Check sheet for the modelled part. Datum: model origin and axes. Units: mm. Round coordinates to 2 decimals unless told otherwise and drop trailing zeros. Write each loop counter-clockwise with the first axis right and the second up, starting at its lowest first coordinate (ties: lowest second). Pieces come first, ordered by that corner, then holes.
Item 1: Cross-section at B-B on x = 111.5. Enter the section's corners in (y, z), plus the area to 3 significant figures.
Item 2: Cross-section at A-A on z = -2.5. Count the separate pieces of the cut face and the enclosed holes in it, plus the area to 3 significant figures.
Item 3: Material ranges on line 1 (Y direction, x = 19, z = -1.5); line 2 (X direction, y = 9, z = -1.9); line 3 (Y direction, x = 10, z = -1.6), recorded low to high.
Item 4: Go/stop test with flat-tipped pins: pin 1 Ø2 at (y, z) = (11.5, -2.5) entering from -X; pin 2 Ø1.5 at (x, z) = (74.5, -1) entering from +Y; pin 3 Ø3 at (x, y) = (10, 0) entering from -Z; pin 4 Ø2 at (y, z) = (-12, -1) entering from +X. Record where each tip stops, or that it passes through.
from build123d import *

# Parameters (mm, degrees)
BRIDA_BASE1_DEPTH     = 4
CROQUIS6_R            = 1.2
CORTAR_EXTRUIR1_DEPTH = 361.432850889
TALADRO_ROSCADO_M3_D  = 2.5
CROQUIS11_R           = 1.7
CORTAR_EXTRUIR2_DEPTH = 361.432850889
REDONDEO1_START       = -5
REDONDEO1_DEPTH       = 6
REDONDEO1_START_2     = -4
REDONDEO1_2_DEPTH     = 4
REDONDEO2_R           = 0.5


with BuildPart() as part:
    # Brida base1: sheet metal written as solids
    # Croquis1 → Brida base1 (new body)
    with BuildSketch(Plane.XY):
        Polygon((0, -4.1), (0, 4.1), (8, 4.1), (15.8, 4.1), (15.8, 17.2), (22.2, 17.2), (22.2, 4.1), (176.8, 4.1), (176.8, 17.2), (183.2, 17.2), (183.2, 4.1), (337.8, 4.1), (337.8, 17.2), (344.2, 17.2), (344.2, 4.1), (352, 4.1), (360, 4.1), (360, -4.1), (352, -4.1), (344.2, -4.1), (344.2, -17.2), (337.8, -17.2), (337.8, -4.1), (183.2, -4.1), (183.2, -17.2), (176.8, -17.2), (176.8, -4.1), (22.2, -4.1), (22.2, -17.2), (15.8, -17.2), (15.8, -4.1), (8, -4.1), align=None)
    extrude(amount=-BRIDA_BASE1_DEPTH)

    # Croquis6 → Cortar-Extruir1 (cut, through all)
    with BuildSketch(Plane.XY):
        with Locations((10, 0)):
            Circle(CROQUIS6_R)
        with Locations((350, 0)):
            Circle(CROQUIS6_R)
        with Locations((170, 0)):
            Circle(CROQUIS6_R)
    extrude(amount=-CORTAR_EXTRUIR1_DEPTH, mode=Mode.SUBTRACT)

    # Taladro roscado M3 (through all)
    with Locations(Plane.XY):
        with Locations((10, 0), (170, 0), (350, 0)):
            Hole(TALADRO_ROSCADO_M3_D / 2)

    # Croquis11 → Cortar-Extruir2 (cut, through all)
    with BuildSketch(Plane.XY):
        with Locations((19, 14)):
            Circle(CROQUIS11_R)
        with Locations((180, 14)):
            Circle(CROQUIS11_R)
        with Locations((341, 14)):
            Circle(CROQUIS11_R)
        with Locations(Location((341, -14, 0), (0, 0, 180))):
            Circle(CROQUIS11_R)
        with Locations(Location((180, -14, 0), (0, 0, 180))):
            Circle(CROQUIS11_R)
        with Locations(Location((19, -14, 0), (0, 0, 180))):
            Circle(CROQUIS11_R)
    extrude(amount=-CORTAR_EXTRUIR2_DEPTH, mode=Mode.SUBTRACT)

    # Redondeo1: read off the stored shape, not the designer's step
    # Redondeo1 outline → Redondeo1 (cut)
    with BuildSketch(Plane.XY.offset(REDONDEO1_START)):
        with BuildLine():
            ThreePointArc((15.8, 14), (16.7372583, 16.2627417), (19, 17.2))
            Line((19, 17.2), (15.8, 17.2))
            Line((15.8, 17.2), (15.8, 14))
        make_face()
        with BuildLine():
            ThreePointArc((19, 17.2), (21.2627417, 16.2627417), (22.2, 14))
            Line((22.2, 14), (22.2, 17.2))
            Line((22.2, 17.2), (19, 17.2))
        make_face()
        with BuildLine():
            ThreePointArc((176.8, 14), (177.7372583, 16.2627417), (180, 17.2))
            Line((180, 17.2), (176.8, 17.2))
            Line((176.8, 17.2), (176.8, 14))
        make_face()
        with BuildLine():
            ThreePointArc((180, 17.2), (182.2627417, 16.2627417), (183.2, 14))
            Line((183.2, 14), (183.2, 17.2))
            Line((183.2, 17.2), (180, 17.2))
        make_face()
        with BuildLine():
            ThreePointArc((337.8, 14), (338.7372583, 16.2627417), (341, 17.2))
            Line((341, 17.2), (337.8, 17.2))
            Line((337.8, 17.2), (337.8, 14))
        make_face()
        with BuildLine():
            ThreePointArc((341, 17.2), (343.2627417, 16.2627417), (344.2, 14))
            Line((344.2, 14), (344.2, 17.2))
            Line((344.2, 17.2), (341, 17.2))
        make_face()
        with BuildLine():
            ThreePointArc((344.2, -14), (343.2627417, -16.2627417), (341, -17.2))
            Line((341, -17.2), (344.2, -17.2))
            Line((344.2, -17.2), (344.2, -14))
        make_face()
        with BuildLine():
            ThreePointArc((341, -17.2), (338.7372583, -16.2627417), (337.8, -14))
            Line((337.8, -14), (337.8, -17.2))
            Line((337.8, -17.2), (341, -17.2))
        make_face()
        with BuildLine():
            ThreePointArc((183.2, -14), (182.2627417, -16.2627417), (180, -17.2))
            Line((180, -17.2), (183.2, -17.2))
            Line((183.2, -17.2), (183.2, -14))
        make_face()
        with BuildLine():
            ThreePointArc((180, -17.2), (177.7372583, -16.2627417), (176.8, -14))
            Line((176.8, -14), (176.8, -17.2))
            Line((176.8, -17.2), (180, -17.2))
        make_face()
        with BuildLine():
            ThreePointArc((22.2, -14), (21.2627417, -16.2627417), (19, -17.2))
            Line((19, -17.2), (22.2, -17.2))
            Line((22.2, -17.2), (22.2, -14))
        make_face()
        with BuildLine():
            ThreePointArc((19, -17.2), (16.7372583, -16.2627417), (15.8, -14))
            Line((15.8, -14), (15.8, -17.2))
            Line((15.8, -17.2), (19, -17.2))
        make_face()
    extrude(amount=REDONDEO1_DEPTH, mode=Mode.SUBTRACT)

    # Redondeo1 2 outline → Redondeo1 2 (add)
    with BuildSketch(Plane.XY.offset(REDONDEO1_START_2)):
        with BuildLine():
            Line((344.2, 4.1), (347.4, 4.1))
            ThreePointArc((347.4, 4.1), (345.1372583, 5.0372583), (344.2, 7.3))
            Line((344.2, 7.3), (344.2, 4.1))
        make_face()
        with BuildLine():
            Line((15.8, 4.1), (15.8, 7.3))
            ThreePointArc((15.8, 7.3), (14.8627417, 5.0372583), (12.6, 4.1))
            Line((12.6, 4.1), (15.8, 4.1))
        make_face()
        with BuildLine():
            Line((22.2, 4.1), (25.4, 4.1))
            ThreePointArc((25.4, 4.1), (23.1372583, 5.0372583), (22.2, 7.3))
            Line((22.2, 7.3), (22.2, 4.1))
        make_face()
        with BuildLine():
            Line((176.8, 4.1), (176.8, 7.3))
            ThreePointArc((176.8, 7.3), (175.8627417, 5.0372583), (173.6, 4.1))
            Line((173.6, 4.1), (176.8, 4.1))
        make_face()
        with BuildLine():
            Line((183.2, 4.1), (186.4, 4.1))
            ThreePointArc((186.4, 4.1), (184.1372583, 5.0372583), (183.2, 7.3))
            Line((183.2, 7.3), (183.2, 4.1))
        make_face()
        with BuildLine():
            Line((337.8, 4.1), (337.8, 7.3))
            ThreePointArc((337.8, 7.3), (336.8627417, 5.0372583), (334.6, 4.1))
            Line((334.6, 4.1), (337.8, 4.1))
        make_face()
        with BuildLine():
            Line((15.8, -4.1), (12.6, -4.1))
            ThreePointArc((12.6, -4.1), (14.8627417, -5.0372583), (15.8, -7.3))
            Line((15.8, -7.3), (15.8, -4.1))
        make_face()
        with BuildLine():
            Line((344.2, -4.1), (344.2, -7.3))
            ThreePointArc((344.2, -7.3), (345.1372583, -5.0372583), (347.4, -4.1))
            Line((347.4, -4.1), (344.2, -4.1))
        make_face()
        with BuildLine():
            Line((337.8, -4.1), (334.6, -4.1))
            ThreePointArc((334.6, -4.1), (336.8627417, -5.0372583), (337.8, -7.3))
            Line((337.8, -7.3), (337.8, -4.1))
        make_face()
        with BuildLine():
            Line((183.2, -4.1), (183.2, -7.3))
            ThreePointArc((183.2, -7.3), (184.1372583, -5.0372583), (186.4, -4.1))
            Line((186.4, -4.1), (183.2, -4.1))
        make_face()
        with BuildLine():
            Line((176.8, -4.1), (173.6, -4.1))
            ThreePointArc((173.6, -4.1), (175.8627417, -5.0372583), (176.8, -7.3))
            Line((176.8, -7.3), (176.8, -4.1))
        make_face()
        with BuildLine():
            Line((22.2, -4.1), (22.2, -7.3))
            ThreePointArc((22.2, -7.3), (23.1372583, -5.0372583), (25.4, -4.1))
            Line((25.4, -4.1), (22.2, -4.1))
        make_face()
    extrude(amount=REDONDEO1_2_DEPTH)

    # Redondeo2
    redondeo2_edges = [part.edges().sort_by_distance(p)[0] for p in [
        (0, -4.1, -2),
        (0, 4.1, -2),
        (360, 4.1, -2),
        (360, -4.1, -2),
    ]]
    fillet(redondeo2_edges, radius=REDONDEO2_R)


solid = part.part
Response values:
1. outline: (-4.1, -4) - (4.1, -4) - (4.1, 0) - (-4.1, 0) - close
1. area: 32.8 mm2
2. separate pieces: 1
2. enclosed holes: 9
2. area: 3,390 mm2
3. line 1: y = -17.2 to -15.7, -12.3 to 12.3, 15.7 to 17.2
3. line 2: x = 15.8 to 22.2, 176.8 to 183.2, 337.8 to 344.2
3. line 3: y = -4.1 to -1.25, 1.25 to 4.1
4. pin 1: stops at x = 15.8
4. pin 2: stops at y = 4.1
4. pin 3: stops at z = -4
4. pin 4: stops at x = 344.2
